Geometry check sheet. Reference: the model listing, model coordinates, mm. Face numbers are marked on the shaded views. A direction names the side the tool comes from. Coordinates: 2 decimals unless noted, no trailing zeros. Loops run counter-clockwise (first coordinate to the right, second up) from the corner with the lowest first, then second, coordinate; pieces in that order, holes last.
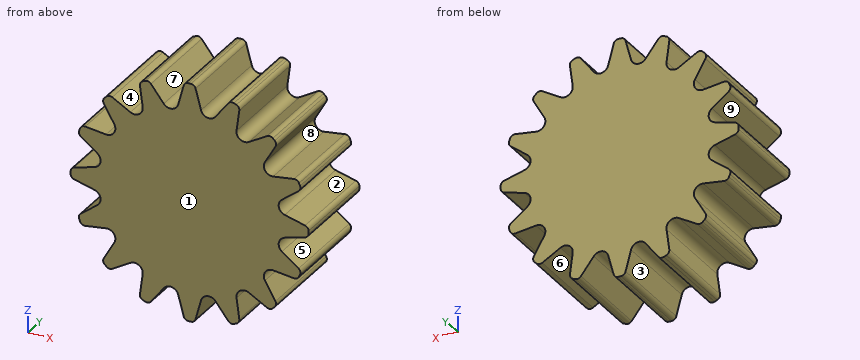
from build123d import *

# Parameters (mm, degrees)
F1_DEPTH = 25.4


with BuildPart() as f1:
    # F0 (on Front) → F1 (new body)
    with BuildSketch(Plane.XZ):
        with BuildLine():
            Line((0.360774, 31.75), (0, 31.75))
            Line((0, 31.75), (-0.360774, 31.75))
            ThreePointArc((-0.360774, 31.75), (-1.133901, 31.487559), (-1.5875, 30.8087))
            Line((-1.5875, 30.8087), (-3.036757, 25.4))
            ThreePointArc((-3.036757, 25.4), (-4.735833, 23.808641), (-6.914562, 24.628657))
            Line((-6.914562, 24.628657), (-10.32332, 29.071037))
            ThreePointArc((-10.32332, 29.071037), (-11.002179, 29.524636), (-11.816887, 29.471237))
            Line((-11.816887, 29.471237), (-12.150199, 29.333175))
            Line((-12.150199, 29.333175), (-12.483511, 29.195113))
            ThreePointArc((-12.483511, 29.195113), (-13.097355, 28.656786), (-13.256638, 27.856018))
            Line((-13.256638, 27.856018), (-12.525757, 22.304424))
            ThreePointArc((-12.525757, 22.304424), (-13.486512, 20.183992), (-15.813201, 20.107824))
            Line((-15.813201, 20.107824), (-20.662509, 22.907573))
            ThreePointArc((-20.662509, 22.907573), (-21.463277, 23.066856), (-22.195534, 22.705746))
            Line((-22.195534, 22.705746), (-22.45064, 22.45064))
            Line((-22.45064, 22.45064), (-22.705746, 22.195534))
            ThreePointArc((-22.705746, 22.195534), (-23.066856, 21.463277), (-22.907573, 20.662509))
            Line((-22.907573, 20.662509), (-20.107824, 15.813201))
            ThreePointArc((-20.107824, 15.813201), (-20.183992, 13.486512), (-22.304424, 12.525757))
            Line((-22.304424, 12.525757), (-27.856018, 13.256638))
            ThreePointArc((-27.856018, 13.256638), (-28.656786, 13.097355), (-29.195113, 12.483511))
            Line((-29.195113, 12.483511), (-29.333175, 12.150199))
            Line((-29.333175, 12.150199), (-29.471237, 11.816887))
            ThreePointArc((-29.471237, 11.816887), (-29.524636, 11.002179), (-29.071037, 10.32332))
            Line((-29.071037, 10.32332), (-24.628657, 6.914562))
            ThreePointArc((-24.628657, 6.914562), (-23.808641, 4.735833), (-25.4, 3.036757))
            Line((-25.4, 3.036757), (-30.8087, 1.5875))
            ThreePointArc((-30.8087, 1.5875), (-31.487559, 1.133901), (-31.75, 0.360774))
            Line((-31.75, 0.360774), (-31.75, 0))
            Line((-31.75, 0), (-31.75, -0.360774))
            ThreePointArc((-31.75, -0.360774), (-31.487559, -1.133901), (-30.8087, -1.5875))
            Line((-30.8087, -1.5875), (-25.4, -3.036757))
            ThreePointArc((-25.4, -3.036757), (-23.808641, -4.735833), (-24.628657, -6.914562))
            Line((-24.628657, -6.914562), (-29.071037, -10.32332))
            ThreePointArc((-29.071037, -10.32332), (-29.524636, -11.002179), (-29.471237, -11.816887))
            Line((-29.471237, -11.816887), (-29.333175, -12.150199))
            Line((-29.333175, -12.150199), (-29.195113, -12.483511))
            ThreePointArc((-29.195113, -12.483511), (-28.656786, -13.097355), (-27.856018, -13.256638))
            Line((-27.856018, -13.256638), (-22.304424, -12.525757))
            ThreePointArc((-22.304424, -12.525757), (-20.183992, -13.486512), (-20.107824, -15.813201))
            Line((-20.107824, -15.813201), (-22.907573, -20.662509))
            ThreePointArc((-22.907573, -20.662509), (-23.066856, -21.463277), (-22.705746, -22.195534))
            Line((-22.705746, -22.195534), (-22.45064, -22.45064))
            Line((-22.45064, -22.45064), (-22.195534, -22.705746))
            ThreePointArc((-22.195534, -22.705746), (-21.463277, -23.066856), (-20.662509, -22.907573))
            Line((-20.662509, -22.907573), (-15.813201, -20.107824))
            ThreePointArc((-15.813201, -20.107824), (-13.486512, -20.183992), (-12.525757, -22.304424))
            Line((-12.525757, -22.304424), (-13.256638, -27.856018))
            ThreePointArc((-13.256638, -27.856018), (-13.097355, -28.656786), (-12.483511, -29.195113))
            Line((-12.483511, -29.195113), (-12.150199, -29.333175))
            Line((-12.150199, -29.333175), (-11.816887, -29.471237))
            ThreePointArc((-11.816887, -29.471237), (-11.002179, -29.524636), (-10.32332, -29.071037))
            Line((-10.32332, -29.071037), (-6.914562, -24.628657))
            ThreePointArc((-6.914562, -24.628657), (-4.735833, -23.808641), (-3.036757, -25.4))
            Line((-3.036757, -25.4), (-1.5875, -30.8087))
            ThreePointArc((-1.5875, -30.8087), (-1.133901, -31.487559), (-0.360774, -31.75))
            Line((-0.360774, -31.75), (0, -31.75))
            Line((0, -31.75), (0.360774, -31.75))
            ThreePointArc((0.360774, -31.75), (1.133901, -31.487559), (1.5875, -30.8087))
            Line((1.5875, -30.8087), (3.036757, -25.4))
            ThreePointArc((3.036757, -25.4), (4.735833, -23.808641), (6.914562, -24.628657))
            Line((6.914562, -24.628657), (10.32332, -29.071037))
            ThreePointArc((10.32332, -29.071037), (11.002179, -29.524636), (11.816887, -29.471237))
            Line((11.816887, -29.471237), (12.150199, -29.333175))
            Line((12.150199, -29.333175), (12.483511, -29.195113))
            ThreePointArc((12.483511, -29.195113), (13.097355, -28.656786), (13.256638, -27.856018))
            Line((13.256638, -27.856018), (12.525757, -22.304424))
            ThreePointArc((12.525757, -22.304424), (13.486512, -20.183992), (15.813201, -20.107824))
            Line((15.813201, -20.107824), (20.662509, -22.907573))
            ThreePointArc((20.662509, -22.907573), (21.463277, -23.066856), (22.195534, -22.705746))
            Line((22.195534, -22.705746), (22.45064, -22.45064))
            Line((22.45064, -22.45064), (22.705746, -22.195534))
            ThreePointArc((22.705746, -22.195534), (23.066856, -21.463277), (22.907573, -20.662509))
            Line((22.907573, -20.662509), (20.107824, -15.813201))
            ThreePointArc((20.107824, -15.813201), (20.183992, -13.486512), (22.304424, -12.525757))
            Line((22.304424, -12.525757), (27.856018, -13.256638))
            ThreePointArc((27.856018, -13.256638), (28.656786, -13.097355), (29.195113, -12.483511))
            Line((29.195113, -12.483511), (29.333175, -12.150199))
            Line((29.333175, -12.150199), (29.471237, -11.816887))
            ThreePointArc((29.471237, -11.816887), (29.524636, -11.002179), (29.071037, -10.32332))
            Line((29.071037, -10.32332), (24.628657, -6.914562))
            ThreePointArc((24.628657, -6.914562), (23.808641, -4.735833), (25.4, -3.036757))
            Line((25.4, -3.036757), (30.8087, -1.5875))
            ThreePointArc((30.8087, -1.5875), (31.487559, -1.133901), (31.75, -0.360774))
            Line((31.75, -0.360774), (31.75, 0))
            Line((31.75, 0), (31.75, 0.360774))
            ThreePointArc((31.75, 0.360774), (31.487559, 1.133901), (30.8087, 1.5875))
            Line((30.8087, 1.5875), (25.4, 3.036757))
            ThreePointArc((25.4, 3.036757), (23.808641, 4.735833), (24.628657, 6.914562))
            Line((24.628657, 6.914562), (29.071037, 10.32332))
            ThreePointArc((29.071037, 10.32332), (29.524636, 11.002179), (29.471237, 11.816887))
            Line((29.471237, 11.816887), (29.333175, 12.150199))
            Line((29.333175, 12.150199), (29.195113, 12.483511))
            ThreePointArc((29.195113, 12.483511), (28.656786, 13.097355), (27.856018, 13.256638))
            Line((27.856018, 13.256638), (22.304424, 12.525757))
            ThreePointArc((22.304424, 12.525757), (20.183992, 13.486512), (20.107824, 15.813201))
            Line((20.107824, 15.813201), (22.907573, 20.662509))
            ThreePointArc((22.907573, 20.662509), (23.066856, 21.463277), (22.705746, 22.195534))
            Line((22.705746, 22.195534), (22.45064, 22.45064))
            Line((22.45064, 22.45064), (22.195534, 22.705746))
            ThreePointArc((22.195534, 22.705746), (21.463277, 23.066856), (20.662509, 22.907573))
            Line((20.662509, 22.907573), (15.813201, 20.107824))
            ThreePointArc((15.813201, 20.107824), (13.486512, 20.183992), (12.525757, 22.304424))
            Line((12.525757, 22.304424), (13.256638, 27.856018))
            ThreePointArc((13.256638, 27.856018), (13.097355, 28.656786), (12.483511, 29.195113))
            Line((12.483511, 29.195113), (12.150199, 29.333175))
            Line((12.150199, 29.333175), (11.816887, 29.471237))
            ThreePointArc((11.816887, 29.471237), (11.002179, 29.524636), (10.32332, 29.071037))
            Line((10.32332, 29.071037), (6.914562, 24.628657))
            ThreePointArc((6.914562, 24.628657), (4.735833, 23.808641), (3.036757, 25.4))
            Line((3.036757, 25.4), (1.5875, 30.8087))
            ThreePointArc((1.5875, 30.8087), (1.133901, 31.487559), (0.360774, 31.75))
        make_face()
    extrude(amount=F1_DEPTH)


solid = f1.part
1) Material ranges on probe 1 along X at (y, z) = (-15.25, 26); probe 2 along X at (y, z) = (-6.5, -22.5); probe 3 along Z at (x, y) = (-21.5, -10), recorded low to high.
Data:
probe 1: x = -13.01 to -7.97, -2.88 to 2.88, 7.97 to 13.01
probe 2: x = -22.4 to -19.96, -12.55 to 12.55, 19.96 to 22.4
probe 3: z = -23.06 to -18.22, -12.57 to 12.57, 18.22 to 23.06
2) Section check A-A on x = -9. Record the cut outline in (y, z), and give its area (3 significant figures).
Data:
outline: (-25.4, -27.35) - (0, -27.35) - (0, 27.35) - (-25.4, 27.35) - close
area: 1,390 mm2
3) Access from +Z, -Z, +X, -X, +Y, -Y to the whole of each face (thin tool, end or side, straight path). Record for the marked faces 5, 6, 7, 8 and 9.
Data:
face 5: +X, +Y, -Y
face 6: -Z, +Y, -Y
face 7: +Z, +Y, -Y
face 8: +Y, -Y
face 9: -X, +Y, -Y
4) Section check B-B on z = -18.5. Record the cut outline in (x, y), and give its area (3 significant figures).
Data:
outline: (-21.66, -25.4) - (21.66, -25.4) - (21.66, 0) - (-21.66, 0) - close
area: 1,100 mm2
5) Mould release check, pull along Z, two halves, no side actions. Record for the marked faces 1, 2, 3 and 4: +Z half, -Z half, draft (parallel to the pull), parting line (faces both ways), or undercut.
Data:
face 1: draft
face 2: undercut
face 3: -Z half
face 4: +Z half
6) Depth check by flat-ended pin: pin 1 (1 mm diameter, centred on y = -17, z = 8.5, fed in from +X); pin 2 (4 mm diameter, centred on x = 18, y = -7, fed in from +Z); pin 3 (3 mm diameter, centred on x = -11, y = -17.5, fed in from +Z). Enter the tip coordinate at first touch or a pass-through.
Data:
pin 1: stops at x = 27.35
pin 2: stops at z = 22.53
pin 3: stops at z = 29.57
